```python
from build123d import *

# Parameters (mm, degrees)
SKETCH1_W           = 20
SKETCH1_H           = 681.33
BOSS_EXTRUDE1_DEPTH = 20
SKETCH2_R           = 2.5
CUT_EXTRUDE1_DEPTH  = 10


with BuildPart() as part:
    # Sketch1 → Boss-Extrude1 (new body)
    with BuildSketch(Plane.XY):
        with Locations((-66.54676259, -268.254928058)):
            Rectangle(SKETCH1_W, SKETCH1_H)
        with Locations((73.45323741, -268.254928058)):
            Rectangle(SKETCH1_W, SKETCH1_H)
        Polygon((-76.54676259, 92.410071942), (-76.54676259, 72.410071942), (-56.54676259, 72.410071942), (63.45323741, 72.410071942), (83.45323741, 72.410071942), (83.45323741, 92.410071942), align=None)
    extrude(amount=BOSS_EXTRUDE1_DEPTH)

    # Sketch2 → Cut-Extrude1 (cut)
    with BuildSketch(Plane(origin=(0, 92.410071942, 0), x_dir=(1, 0, 0), z_dir=(0, 1, 0))):
        with Locations(Location((48.45323741, -10, 0), (0, 0, 180))):
            Circle(SKETCH2_R)
    extrude(amount=-CUT_EXTRUDE1_DEPTH, mode=Mode.SUBTRACT)


solid = part.part
```
Read the model definition and answer for the solid it produces. Units are mm, in the model's axes. A direction names the side the tool comes from. Give positions to 0.01 mm unless a question says otherwise; leave off trailing zeros. Write each loop counter-clockwise with the first axis right and the second up, starting at its lowest first coordinate (ties: lowest second). Pieces come first, ordered by that corner, then holes. Notation, with made-up numbers: M 27.5,-34.5 L 33.5,-34.5 A11 cw 33.5,-25.5 Z; hole C 56.5,71 d11. An arc over 180 degrees is marked long. Put each result on its own line as item: value. Start each with the question number.
1. The part is cut by section B-B, the plane z = 3. Give the vertices of the cut face in (x, y).
2. The part is cut by section A-A, the plane y = -40.5. Give the vertices of the cut face in (x, z), and give its area (3 significant figures).
3. Which of the six approach directions +Z, -Z, +X, -X, +Y, -Y give full straight-line access (tool end or side, diameter ignored) to faces 4 (the flat face through (63.453, -273, 10)), 5 (the flat face through (5, 92.41, 10))?
4. For a pull along X with two mould halves and no side action, classify faces 1 (the flat face through (83.453, -263, 10)), 2 (the flat face through (3, 72.41, 10)), 3 (the flat face through (73, -608.92, 10)) as released by +X, released by -X, zero draft, split by the parting line, or undercut.
5. The part is cut by section C-C, the plane x = -17.5. Give the vertices of the cut face in (y, z), and give its area (3 significant figures).
6. Consider line 1 along X through (y, z) = (-22.5, 5.5); line 2 along Y through (x, z) = (26, 15). Determine where each line is inside the solid, lowest interval first.
7. Each of these flat-tipped pins is pushed along its axis until it touches: pin 1 Ø6 at (x, z) = (-21.5, 11.5) entering from -Y; pin 2 Ø1.5 at (x, z) = (48, 11) entering from +Y. Where does it stop, or does it pass through?
Final values:
1. outline: M -76.55,-608.92 L -56.55,-608.92 L -56.55,72.41 L 63.45,72.41 L 63.45,-608.92 L 83.45,-608.92 L 83.45,92.41 L -76.55,92.41 Z
2. outline: M -76.55,0 L -56.55,0 L -56.55,20 L -76.55,20 Z; M 63.45,0 L 83.45,0 L 83.45,20 L 63.45,20 Z
2. area: 800 mm²
3. face 4: +Z, -Z, -Y
3. face 5: +Z, -Z, +X, -X, +Y
4. face 1: released by +X
4. face 2: undercut
4. face 3: zero draft
5. outline: M 72.41,0 L 92.41,0 L 92.41,20 L 72.41,20 Z
5. area: 400 mm²
6. line 1: x = -76.55 to -56.55, 63.45 to 83.45
6. line 2: y = 72.41 to 92.41
7. pin 1: stops at y = 72.41
7. pin 2: stops at y = 82.41
